Autodesk Inventor part; units mm, degrees
ref_plane "Work Plane2" through (0, 0, -127) normal (0, 0, -1) x (-1, 0, 0)
ref_plane "YZ Plane" through (0, 0, 0) normal (1, 0, 0) x (0, 1, 0)
ref_plane "XZ Plane" through (0, 0, 0) normal (0, 1, 0) x (-1, 0, 0)
sketch "Sketch3" plane through (0, 0, 0) normal (0, 0, 1) x (1, 0, 0)
  circle A0 centre (0, 0) radius 4.5
  dimension "d5" = 9
extrude "Extrusion3" add sketch "Sketch3" along normal blind 114.3
ref_plane "Work Plane2" through (0, 0, -127) normal (0, 0, -1) x (-1, 0, 0)
mirror "Mirror1" about plane through (0, 0, -127) normal (0, 0, -1) of "Extrusion3"
sketch "Sketch5" plane through (0, 0, -127) normal (0, 0, -1) x (-1, 0, 0)
  circle A0 centre (0, 0) radius 4.5
extrude "Extrusion4" add sketch "Sketch5" along normal mid plane 254
sketch "Sketch6" plane through (0, 0, 114.3) normal (0, 0, 1) x (1, 0, 0)
  circle A0 centre (0, 0) radius 4.5
extrude "Extrusion5" add sketch "Sketch6" along normal blind 121.92
sketch "Sketch7" plane through (0, 0, -368.3) normal (0, 0, -1) x (-1, 0, 0)
  circle A0 centre (0, 0) radius 4.5
extrude "Extrusion6" add sketch "Sketch7" along normal blind 121.92
thread "Thread3"
thread "Thread4"
properties part number "Axle"
Geometry: final body of the model. Coordinates: model frame, mm. Round coordinates to 2 decimals unless told otherwise and drop trailing zeros. Write each loop counter-clockwise with the first axis right and the second up, starting at its lowest first coordinate (ties: lowest second). Pieces come first, ordered by that corner, then holes.
Item 1: Section query A-A (z = 103.5). Return loops of the section in (x, y).
Item 2: Section query B-B (y = -1.5). Return loops of the section in (x, z).
Item 3: Pin query (flat end, axial travel): P1, Ø1, axis at x = 2.5, z = 29, coming from the -Y side; P2, Ø3, axis at y = 3, z = -178, coming from the +X side. Return the tip coordinate at first contact, or that it passes through.
Item 4: Material intervals for L1, parallel to Y at x = -0.75, z = 119; L2, parallel to Y at x = 2.5, z = -219, sorted ascending.
Item 5: Section query C-C (x = 1.75). Return loops of the section in (y, z).
Completed:
1. outline: circle Ø9 at (0, 0)
2. outline: (-4.24, -490.22) - (4.24, -490.22) - (4.24, 236.22) - (-4.24, 236.22) - close
3. P1: stops at y = -4.03
3. P2: stops at x = 4.24
4. L1: y = -4.44 to 4.44
4. L2: y = -3.74 to 3.74
5. outline: (-4.15, -490.22) - (4.15, -490.22) - (4.15, 236.22) - (-4.15, 236.22) - close
